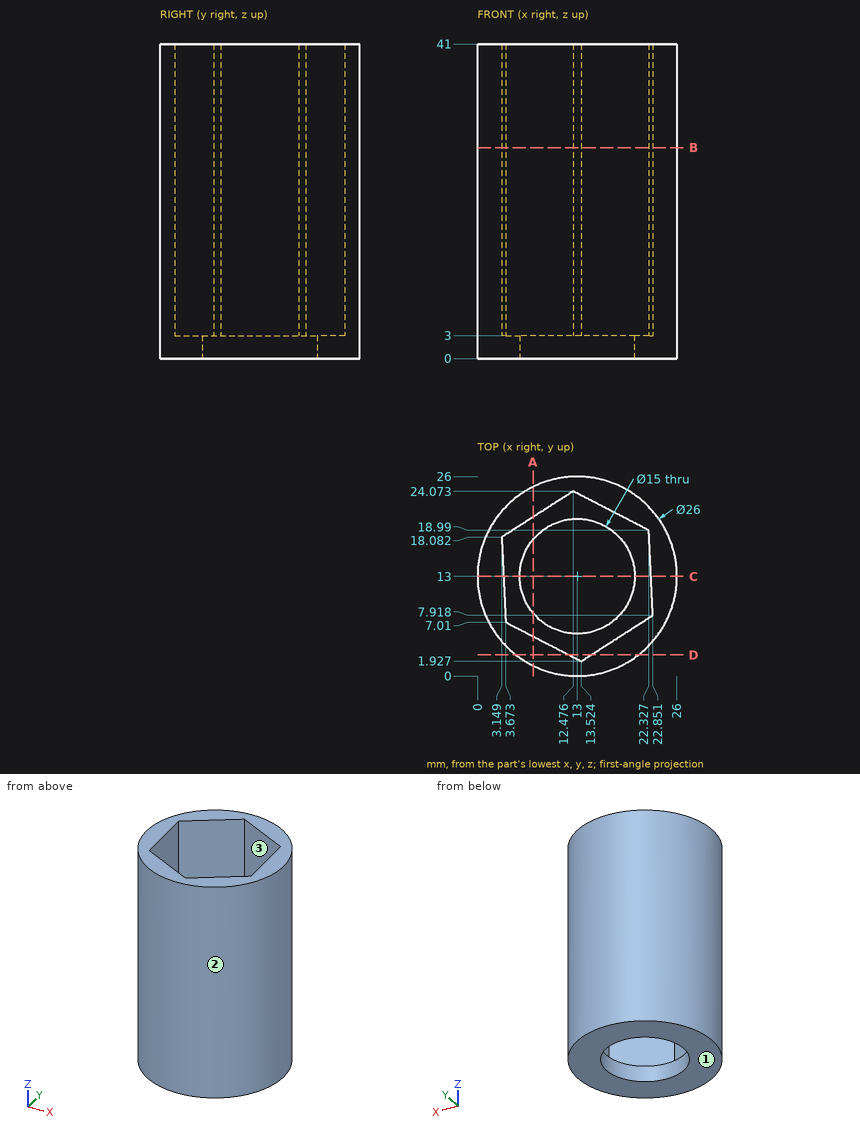
Geometry check sheet. Reference: drawing and pictorial views, mm from the part's lowest x, y, z. Coordinates: 2 decimals unless noted, no trailing zeros. Order: outer loops, then holes, each group sorted by start corner. A loop starts at its lowest first (then second) coordinate and runs counter-clockwise, first axis right, second up. Notation, with made-up numbers: (52, 12) -> (110, 12) arc R26 ccw to (110, 31) -> close; hole circle Ø1 at (63.25, -40). An arc over 180 degrees is marked (long way). Put each result on its own line as item: value. Start each with the question number.
1) Cross-section at C-C (y = 13). Enter the section's corners in (x, z).
2) Go/stop test with flat-tipped pins: pin 1 (6 mm diameter, centred on y = 4, z = 17.5, fed in from -X); pin 2 (8 mm diameter, centred on x = 17.5, y = 15.5, fed in from +Z); pin 3 (6 mm diameter, centred on y = 9, z = 14.5, fed in from -X); pin 4 (12 mm diameter, centred on x = 13, y = 13, fed in from +Z). Record where each tip stops, or that it passes through.
3) Cross-section at A-A (x = 7.25). Enter the section's corners in (y, z) (1 decimal).
4) Cross-section at B-B (z = 27.5). Enter the section's corners in (x, y) (1 decimal).
5) Release check for a two-part mould opening along Y. For the marked faces 1, 2 and 3 record: pulls with the +Y half, pulls with the -Y half, needs draft (parallel to the pull), parting line crosses it, or undercut.
6) Cross-section at D-D (y = 2.75). Enter the section's corners in (x, z) (1 decimal).
7) Material ranges on L1, parallel to Y at x = 13, z = 2.3; L2, parallel to Z at x = 8.5, y = 21; L3, parallel to X at y = 9.75, z = 30 (1 decimal), recorded low to high.
Geometry check:
1. outline: (0, 0) -> (5.5, 0) -> (5.5, 3) -> (3.39, 3) -> (3.39, 41) -> (0, 41) -> close; (20.5, 0) -> (26, 0) -> (26, 41) -> (22.61, 41) -> (22.61, 3) -> (20.5, 3) -> close
2. pin 1: stops at x = 1.47
2. pin 2: stops at z = 3
2. pin 3: stops at x = 0.04
2. pin 4: passes through
3. outline: (1.3, 0) -> (8.2, 0) -> (8.2, 3) -> (5.2, 3) -> (5.2, 41) -> (1.3, 41) -> close; (17.8, 0) -> (24.7, 0) -> (24.7, 41) -> (20.7, 41) -> (20.7, 3) -> (17.8, 3) -> close
4. outline: circle Ø26 at (13, 13); hole (3.1, 18.1) -> (3.7, 7) -> (13.5, 1.9) -> (22.9, 7.9) -> (22.3, 19) -> (12.5, 24.1) -> close
5. face 1: needs draft
5. face 2: parting line crosses it
5. face 3: undercut
6. outline: (5, 0) -> (21, 0) -> (21, 41) -> (14.8, 41) -> (14.8, 3) -> (11.9, 3) -> (11.9, 41) -> (5, 41) -> close
7. L1: y = 0 to 5.5, 20.5 to 26
7. L2: z = 0 to 3
7. L3: x = 0.4 to 3.5, 22.8 to 25.6
